from build123d import *

# Parameters (mm, degrees)
SKETCH_W        = 30
SKETCH_H        = 28
PAD_DEPTH       = 4
SKETCH001_W     = 4
SKETCH001_H     = 28
PAD001_DEPTH    = 6
PAD001_FACE5_W  = 28
PAD001_FACE5_H  = 4
PAD002_DEPTH    = 4
SKETCH002_W     = 28
SKETCH002_H     = 4
PAD003_DEPTH    = 40
SKETCH003_R     = 2.5
POCKET_DEPTH    = 5
SKETCH004_R     = 1.65
POCKET001_DEPTH = 5
SKETCH005_W     = 4
SKETCH005_H     = 28
PAD004_DEPTH    = 10
SKETCH006_W     = 28
SKETCH006_H     = 4
PAD005_DEPTH    = 25
FILLET_R        = 1
CHAMFER_SIZE    = 1


with BuildPart() as part:
    # Sketch → Pad (new body)
    with BuildSketch(Plane.XY):
        with Locations((0, -14)):
            Rectangle(SKETCH_W, SKETCH_H)
    extrude(amount=PAD_DEPTH)

    # Sketch001 (on Face6 of Pad) → Pad001 (join)
    with BuildSketch(Plane.XY.offset(4)):
        with Locations((13, -14)):
            Rectangle(SKETCH001_W, SKETCH001_H)
    extrude(amount=PAD001_DEPTH)

    # Pad001 Face5 → Pad002 (add)
    with BuildSketch(Plane(origin=(13, -14, 10), x_dir=(0, 1, 0), z_dir=(0, 0, 1))):
        Rectangle(PAD001_FACE5_W, PAD001_FACE5_H)
    extrude(amount=PAD002_DEPTH)

    # Sketch002 (on Face8 of Pad002) → Pad003 (join)
    with BuildSketch(Plane.YZ.offset(15)):
        with Locations((-14, 12)):
            Rectangle(SKETCH002_W, SKETCH002_H)
    extrude(amount=PAD003_DEPTH)

    # Sketch003 (on Face10 of Pad003) → Pocket (cut)
    with BuildSketch(Plane.XY.offset(14)):
        with Locations((25, -5)):
            Circle(SKETCH003_R)
        with Locations((25, -23)):
            Circle(SKETCH003_R)
        with Locations((45, -5)):
            Circle(SKETCH003_R)
        with Locations((45, -23)):
            Circle(SKETCH003_R)
    extrude(amount=-POCKET_DEPTH, mode=Mode.SUBTRACT)

    # Sketch004 (on Face5 of Pocket) → Pocket001 (cut)
    with BuildSketch(Plane.XY.offset(4)):
        with Locations((7, -8)):
            Circle(SKETCH004_R)
        with Locations((7, -19)):
            Circle(SKETCH004_R)
    extrude(amount=-POCKET001_DEPTH, mode=Mode.SUBTRACT)

    # Sketch005 (on Face4 of Pocket001) → Pad004 (join)
    with BuildSketch(Plane(origin=(0, 0, 0), x_dir=(1, 0, 0), z_dir=(0, 0, -1))):
        with Locations((13, 14)):
            Rectangle(SKETCH005_W, SKETCH005_H)
    extrude(amount=PAD004_DEPTH)

    # Sketch006 (on Face18 of Pad004) → Pad005 (join)
    with BuildSketch(Plane.YZ.offset(15)):
        with Locations((-14, -8)):
            Rectangle(SKETCH006_W, SKETCH006_H)
    extrude(amount=PAD005_DEPTH)

    # Fillet
    fillet_edges = [part.edges().sort_by_distance(p)[0] for p in [
        (15, -14, 10),
        (15, -14, -6),
        (11, -14, 4),
        (11, -14, 0),
        (-15, 0, 2),
        (-15, -28, 2),
        (11, -14, 14),
        (11, -14, -10),
    ]]
    fillet(fillet_edges, radius=FILLET_R)

    # Chamfer
    chamfer_edges = [part.edges().sort_by_distance(p)[0] for p in [
        (40, -14, -6),
        (55, -14, 10),
        (40, -14, -10),
        (55, -14, 14),
    ]]
    chamfer(chamfer_edges, length=CHAMFER_SIZE)


solid = part.part
Geometry: final body of the model. Coordinates: model frame, mm. A direction names the side the tool comes from. Round coordinates to 2 decimals unless told otherwise and drop trailing zeros. Loops run counter-clockwise (first coordinate to the right, second up) from the corner with the lowest first, then second, coordinate; pieces in that order, holes last. Notation, with made-up numbers: M -37,66 L 17,66 A26 cw 17,92 Z; hole C 37,61.5 d8. An arc over 180 degrees is marked long. Put each result on its own line as item: value. Start each with the question number.
(1) Section query B-B (x = 25). Return loops of the section in (y, z).
(2) Draft query along Y for faces 4 (the face through (24.67, -20.52, 12.03)), 5 (the face through (13, -28, 3)), 6 (the face through (33, -14, 14)). Return one class per face: +Y half, -Y half, draft (parallel to the pull), parting line (faces both ways), or undercut.
(3) Section query A-A (y = -5). State how many separate pieces and enclosed holes the cut face has, then the cut area to 3 significant figures.
(4) Section query D-D (y = -15). Return loops of the section in (x, z), then the cut area to 3 significant figures.
(5) Set-up query: faces 1 (the face through (23.16, -3.31, 12.03)), 2 (the face through (27, -14, -6)), 3 (the face through (11, -14, 9)). Return all of +Z, -Z, +X, -X, +Y, -Y with unobstructed straight access to the full face (end or side cutting, diameter ignored); none if empty.
(6) Contact query for flat-ended pins moving along their axis: pin 1 Ø4 at (y, z) = (-14, -5) entering from -X; pin 2 Ø2 at (y, z) = (-9.5, -8) entering from +X; pin 3 Ø8 at (x, y) = (45, -5) entering from -Z. Output: stop coordinate, or through.
(7) Material intervals for line 1 along Y through (x, z) = (45, 11.5); line 2 along Y through (x, z) = (7, 3); line 3 along Z through (x, y) = (16, -18), sorted ascending. Write a range as [from, to].
(8) Section query C-C (x = 7). Return loops of the section in (y, z), then the cut area to 3 significant figures.
Findings below:
1. outline: M -28,-10 L 0,-10 L 0,-6 L -28,-6 Z; M -28,10 L -25.5,10 L -25.5,14 L -28,14 Z; M -20.5,10 L -7.5,10 L -7.5,14 L -20.5,14 Z; M -2.5,10 L 0,10 L 0,14 L -2.5,14 Z
2. face 4: undercut
2. face 5: -Y half
2. face 6: draft
3. separate pieces: 3
3. enclosed holes: 0
3. area: 418 mm2
4. outline: M -15,0 L 10,0 A1 cw 11,-1 L 11,-9 A1 ccw 12,-10 L 39,-10 L 40,-9 L 40,-7 L 39,-6 L 16,-6 A1 cw 15,-5 L 15,9 A1 cw 16,10 L 54,10 L 55,11 L 55,13 L 54,14 L 12,14 A1 ccw 11,13 L 11,5 A1 cw 10,4 L -15,4 Z
4. area: 458 mm2
5. face 1: +Z
5. face 2: +X, +Y, -Y
5. face 3: +Z, -X, +Y, -Y
6. pin 1: stops at x = 11
6. pin 2: stops at x = 40
6. pin 3: stops at z = 10
7. line 1: y = [-28, -25.5], [-20.5, -7.5], [-2.5, 0]
7. line 2: y = [-28, -20.65], [-17.35, -9.65], [-6.35, 0]
7. line 3: z = [-10, -6], [10, 14]
8. outline: M -28,0 L -20.65,0 L -20.65,4 L -28,4 Z; M -17.35,0 L -9.65,0 L -9.65,4 L -17.35,4 Z; M -6.35,0 L 0,0 L 0,4 L -6.35,4 Z
8. area: 85.6 mm2
